The model under review builds one solid part; all positions refer to its coordinate system, in mm. A direction names the side the tool comes from. Round coordinates to 2 decimals unless told otherwise and drop trailing zeros. Write each loop counter-clockwise with the first axis right and the second up, starting at its lowest first coordinate (ties: lowest second). Pieces come first, ordered by that corner, then holes.
Item 1: Add section A-A (z = 0). Give the boundary of the cut face in (x, y).
Item 2: Add section C-C (y = -2.25). Give the boundary of the cut face in (x, z), plus the area to 3 significant figures.
Item 3: Draft analysis for pull direction Z (two halves, no side actions). For faces 3 (the face through (13.507, -7.493, -0.33)), 4 (the face through (1.76, -0.16, 4.87)), 5 (the face through (1.76, 4.87, 0.16)), state which applies: +Z half, -Z half, draft (parallel to the pull), parting line (faces both ways), or undercut.
Item 4: To check wall thickness, follow L1, parallel to X at y = 0, z = 4.2; L2, parallel to X at y = -1, z = -7; L3, parallel to Z at x = 7.5, y = 0. State the ranges of each line that lie inside material, in increasing order.
Item 5: Add section D-D (x = 3). Give the boundary of the cut face in (y, z).
Item 6: Clearance check with flat-ended pins moving along their axes: pin 1 Ø1.5 at (x, y) = (3, 0) entering from +Z; pin 2 Ø4 at (x, y) = (6, -2.5) entering from -Z; pin 3 Ø4 at (y, z) = (0, 0) entering from +X; pin 4 Ø1.5 at (x, y) = (5.5, 3) entering from -Z. State where each tip first meets the part, or that it passes through.
Item 7: Machinability: for faces 1 (the face through (9.549, -6.094, -0.268)), 2 (the face through (14, -2, -2)), which of the approach directions +Z, -Z, +X, -X, +Y, -Y give a long, thin tool a straight path to every point of the face, cutting with its end or side? Answer none if there is none.
```python
from build123d import *

# Parameters (mm, degrees)
SKETCH2_W = 1.25
SKETCH2_H = 7.5
SKETCH4_W = 1.25
SKETCH4_H = 7.5


with BuildPart() as part:
    # Sketch1 → Revolve1 (revolve)
    with BuildSketch(Plane.XY):
        Polygon((0, 2.5), (0, 7.5), (6, 7.5), (6, 6.1), (13, 6.1), (13, 7.5), (14, 7.5), (14, 2.5), align=None)
    revolve(axis=Axis((0, 0, 0), (-1, 0, 0)))

    # Sketch2 → M3x0.5 Tapped Hole1 (revolve, cut)
    with BuildSketch(Plane(origin=(3, 0, 0), x_dir=(0, 0, -1), z_dir=(1, 0, 0))):
        with Locations((0.625, 3.75)):
            Rectangle(SKETCH2_W, SKETCH2_H)
    revolve(axis=Axis((3, -6.35, 0), (0, 1, 0)), mode=Mode.SUBTRACT)

    # Sketch4 → M3x0.5 Tapped Hole2 (revolve, cut)
    with BuildSketch(Plane.YZ.offset(3)):
        with Locations((0.625, 3.75)):
            Rectangle(SKETCH4_W, SKETCH4_H)
    revolve(axis=Axis((3, 0, -6.35), (0, 0, 1)), mode=Mode.SUBTRACT)


solid = part.part
```
Numbers:
1. outline: (0, -7.5) - (6, -7.5) - (6, -6.1) - (13, -6.1) - (13, -7.5) - (14, -7.5) - (14, -2.5) - (0, -2.5) - close; (0, 2.5) - (1.75, 2.5) - (1.75, 7.5) - (0, 7.5) - close; (4.25, 2.5) - (14, 2.5) - (14, 7.5) - (13, 7.5) - (13, 6.1) - (6, 6.1) - (6, 7.5) - (4.25, 7.5) - close
2. outline: (0, -7.15) - (6, -7.15) - (6, -5.67) - (13, -5.67) - (13, -7.15) - (14, -7.15) - (14, -1.09) - (0, -1.09) - close; (0, 1.09) - (14, 1.09) - (14, 7.15) - (13, 7.15) - (13, 5.67) - (6, 5.67) - (6, 7.15) - (0, 7.15) - close
2. area: 149 mm2
3. face 3: parting line
3. face 4: draft
3. face 5: undercut
4. L1: x = 0 to 1.75, 4.25 to 14
4. L2: x = 0 to 6, 13 to 14
4. L3: z = -6.1 to -2.5, 2.5 to 6.1
5. outline: (-1.25, 2.17) - (-1.25, 7.4) arc R7.5 ccw (long way) to (7.4, -1.25) - (2.17, -1.25) arc R2.5 cw (long way) to start; (1.25, 2.17) arc R2.5 cw to (2.17, 1.25) - (7.4, 1.25) arc R7.5 ccw to (1.25, 7.4) - close
6. pin 1: stops at z = -2.38
6. pin 2: stops at z = -7.48
6. pin 3: passes through
6. pin 4: stops at z = -7.15
7. face 1: none
7. face 2: +Z, -Z, +X, +Y, -Y
